from build123d import *

# Parameters (mm, degrees)
BOSS_EXTRUDE1_DEPTH = 4


with BuildPart() as part:
    # Sketch1 → Boss-Extrude1 (new body)
    with BuildSketch(Plane.YZ):
        Polygon((37.5, -50), (352.5, -50), (390, 0), (390, 150), (0, 150), (0, 0), align=None)
        with BuildLine():
            ThreePointArc((339.15, 117.1), (341.25, 115), (343.35, 117.1))
            Line((343.35, 117.1), (343.35, 142.9))
            ThreePointArc((343.35, 142.9), (341.25, 145), (339.15, 142.9))
            Line((339.15, 142.9), (339.15, 117.1))
        make_face(mode=Mode.SUBTRACT)
        with BuildLine():
            ThreePointArc((144.15, 117.1), (146.25, 115), (148.35, 117.1))
            Line((148.35, 117.1), (148.35, 142.9))
            ThreePointArc((148.35, 142.9), (146.25, 145), (144.15, 142.9))
            Line((144.15, 142.9), (144.15, 117.1))
        make_face(mode=Mode.SUBTRACT)
        with BuildLine():
            Line((50.85, 142.9), (50.85, 117.1))
            ThreePointArc((50.85, 117.1), (48.75, 115), (46.65, 117.1))
            Line((46.65, 117.1), (46.65, 142.9))
            ThreePointArc((46.65, 142.9), (48.75, 145), (50.85, 142.9))
        make_face(mode=Mode.SUBTRACT)
        with BuildLine():
            Line((245.85, 142.9), (245.85, 117.1))
            ThreePointArc((245.85, 117.1), (243.75, 115), (241.65, 117.1))
            Line((241.65, 117.1), (241.65, 142.9))
            ThreePointArc((241.65, 142.9), (243.75, 145), (245.85, 142.9))
        make_face(mode=Mode.SUBTRACT)
    extrude(amount=BOSS_EXTRUDE1_DEPTH)


solid = part.part
For this review, take the finished solid that the model builds, in its own axes (mm). Round coordinates to 2 decimals unless told otherwise and drop trailing zeros. Write each loop counter-clockwise with the first axis right and the second up, starting at its lowest first coordinate (ties: lowest second). Pieces come first, ordered by that corner, then holes. Notation, with made-up numbers: (-28, 39) - (0, 39) arc R21 cw to (0, 49) - close; hole circle Ø8 at (27.25, 64). An arc over 180 degrees is marked (long way). Write item = value, one per line. Start each with the question number.
1. Consider section C-C on z = -20. State the section outline as (x, y) points.
2. Consider section A-A on z = 121. State the section outline as (x, y) points.
3. For pin 1 Ø1.5 at (x, z) = (2, -22) entering from +Y, flat-tipped, find the tip position at first contact; note if it passes through.
4. Consider section D-D on y = 32.5. State the section outline as (x, z) points, plus the area to 3 significant figures.
5. Consider section B-B on x = 3.25. State the section outline as (y, z) points.
6. Wall thickness on L1, parallel to Y at x = 2.25, z = 138; L2, parallel to Y at x = 2.9, z = -32; L3, parallel to Y at x = 2.25, z = -10: over which ranges is each line inside the solid? List them lowest first.
Evaluation:
q1.outline = (0, 15) - (4, 15) - (4, 375) - (0, 375) - close
q2.outline = (0, 0) - (4, 0) - (4, 46.65) - (0, 46.65) - close; (0, 50.85) - (4, 50.85) - (4, 144.15) - (0, 144.15) - close; (0, 148.35) - (4, 148.35) - (4, 241.65) - (0, 241.65) - close; (0, 245.85) - (4, 245.85) - (4, 339.15) - (0, 339.15) - close; (0, 343.35) - (4, 343.35) - (4, 390) - (0, 390) - close
q3.pin_1 = 374.06
q4.outline = (0, -43.33) - (4, -43.33) - (4, 150) - (0, 150) - close
q4.area = 773 mm2
q5.outline = (0, 0) - (37.5, -50) - (352.5, -50) - (390, 0) - (390, 150) - (0, 150) - close; hole (46.65, 117.1) arc R2.1 ccw to (50.85, 117.1) - (50.85, 142.9) arc R2.1 ccw to (46.65, 142.9) - close; hole (144.15, 117.1) arc R2.1 ccw to (148.35, 117.1) - (148.35, 142.9) arc R2.1 ccw to (144.15, 142.9) - close; hole (241.65, 117.1) arc R2.1 ccw to (245.85, 117.1) - (245.85, 142.9) arc R2.1 ccw to (241.65, 142.9) - close; hole (339.15, 117.1) arc R2.1 ccw to (343.35, 117.1) - (343.35, 142.9) arc R2.1 ccw to (339.15, 142.9) - close
q6.L1 = 0 to 46.65, 50.85 to 144.15, 148.35 to 241.65, 245.85 to 339.15, 343.35 to 390
q6.L2 = 24 to 366
q6.L3 = 7.5 to 382.5
